Build history of the part. All positions in model axes, mm. A direction names the side the tool comes from. Give positions to 0.01 mm unless a question says otherwise; leave off trailing zeros. Write each loop counter-clockwise with the first axis right and the second up, starting at its lowest first coordinate (ties: lowest second). Pieces come first, ordered by that corner, then holes. Notation, with made-up numbers: (4, -31) -> (42, -31) arc R24 cw to (42, 5) -> close; hole circle Ø6 at (-29, 76.5). An arc over 180 degrees is marked (long way). Put each result on its own line as item: value.
Autodesk Inventor part; units mm, degrees
ref_plane "YZ Plane" through (0, 0, 0) normal (1, 0, 0) x (0, 1, 0)
ref_plane "XZ Plane" through (0, 0, 0) normal (0, 1, 0) x (-1, 0, 0)
ref_plane "XY Plane" through (0, 0, 0) normal (0, 0, 1) x (1, 0, 0)
sketch "Sketch1" plane through (0, 0, 0) normal (0, 0, 1) x (1, 0, 0)
  line L0 (65, -65) -> (-65, -65)
  line L1 (-65, -65) -> (-65, 65)
  line L2 (-65, 65) -> (65, 65)
  line L3 (65, 65) -> (65, -65)
  line L4 (65, -65) -> (-65, 65) construction
  line L5 (-65, -65) -> (65, 65) construction
  circle A0 centre (0, 0) radius 72.5 construction
  circle A1 centre (-51.2652, 51.2652) radius 4.5
  circle A2 centre (51.2652, 51.2652) radius 4.5
  line L6 (-65, 0) -> (65, 0) construction
  circle A3 centre (-51.2652, -51.2652) radius 4.5
  circle A4 centre (51.2652, -51.2652) radius 4.5
  dimension "d0" = 130
  dimension "d1" = 130
  dimension "d2" = 145
  dimension "d3" = 9
  dimension "d4" = 9
extrude "Extrusion1" add sketch "Sketch1" along normal blind 10
fillet "Fillet1" radius 5 4 edges at (-65, -65, 5) (65, -65, 5) (65, 65, 5) (-65, 65, 5)
sketch "Sketch2" plane through (0, 0, 10) normal (0, 0, 1) x (1, 0, 0)
  circle A0 centre (0, 0) radius 55
  circle A1 centre (0, 0) radius 54
  dimension "d8" = 110
extrude "Extrusion2" add sketch "Sketch2" along normal blind 5
sketch "Sketch3" plane through (0, 0, 10) normal (0, 0, 1) x (1, 0, 0)
  circle A0 centre (0, 0) radius 15
  line L0 (0, 0) -> (24.7487, -24.7487) construction
  line L1 (0, 0) -> (35, 0) construction
  line L2 (0, 0) -> (-24.7487, -24.7487) construction
  line L3 (0, 0) -> (35, 0) construction
  line L4 (0, 0) -> (24.7487, 24.7487) construction
  line L5 (0, 0) -> (-24.7487, 24.7487) construction
  line L6 (0.7071, 0.7071) -> (-24.0416, 25.4558) construction
  line L7 (37.8235, -36.4093) -> (25.4457, -24.0315)
  line L8 (36.4093, -37.8235) -> (24.0315, -25.4457)
  line L9 (-36.4093, -37.8235) -> (-24.0315, -25.4457)
  line L10 (-37.8235, -36.4093) -> (-25.4457, -24.0315)
  line L11 (-25.4457, 24.0315) -> (-37.8235, 36.4093)
  line L12 (-24.0315, 25.4457) -> (-36.4093, 37.8235)
  line L13 (-25.4457, 24.0315) -> (-25.4558, 24.0416)
  line L14 (-24.0315, 25.4457) -> (-24.0416, 25.4558)
  line L15 (-25.4457, 24.0315) -> (-25.4558, 24.0416)
  line L16 (36.4093, 37.8235) -> (24.0315, 25.4457)
  line L17 (37.8235, 36.4093) -> (25.4457, 24.0315)
  arc A1 (-24.0315, -25.4457) -> (24.0315, -25.4457) centre (0, 0) ccw
  arc A2 (-25.4457, 24.0315) -> (-25.4457, -24.0315) centre (0, 0) ccw
  arc A3 (25.4457, -24.0315) -> (25.4457, 24.0315) centre (0, 0) ccw
  arc A4 (24.0315, 25.4457) -> (-24.0315, 25.4457) centre (0, 0) ccw
  arc A5 (-36.4093, -37.8235) -> (36.4093, -37.8235) centre (0, 0) ccw
  arc A6 (-37.8235, 36.4093) -> (-37.8235, -36.4093) centre (0, 0) ccw
  arc A7 (37.8235, -36.4093) -> (37.8235, 36.4093) centre (0, 0) ccw
  arc A8 (36.4093, 37.8235) -> (-36.4093, 37.8235) centre (0, 0) ccw
  circle A9 centre (0, 0) radius 54
  dimension "d12" = 30
  dimension "d14" = 45
  dimension "d15" = 135
extrude "Extrusion3" add sketch "Sketch3" along normal blind 5
sketch "Sketch4" plane through (0, 0, 0) normal (0, 1, 0) x (-1, 0, 0)
  line L0 (15, 15) -> (15, 10)
  line L1 (15, 10) -> (15, 15)
  line L2 (0, 15) -> (11, 15) construction
  line L3 (15, 15) -> (13, 15)
  line L4 (13, 15) -> (13, 20)
  line L5 (11, 16) -> (11, 67) construction
  line L6 (60, 10) -> (65, 10) construction
  line L7 (13, 20) -> (11, 20)
  line L8 (11, 67) -> (11, 20)
  line L9 (11, 67) -> (0, 67)
  line L10 (0, 67) -> (0, 10)
  line L11 (15, 10) -> (0, 10)
  line L12 (0, -13.4) -> (0, 80.4)
  point P0 (0, 0)
  dimension "d18" = 11
  dimension "d19" = 2
  dimension "d20" = 5
  dimension "d21" = 57
revolve "Revolution1" add sketch "Sketch4" angle 360 about axis through (0, 0, -10) along (0, 0, 1)
sketch "Sketch5" plane through (0, 0, 0) normal (0, 0, -1) x (-1, 0, 0)
  line L0 (-45.7652, 55.7652) -> (45.7652, 55.7652)
  line L1 (55.7652, 45.7652) -> (55.7652, -45.7652)
  line L2 (45.7652, -55.7652) -> (-45.7652, -55.7652)
  line L3 (-55.7652, -45.7652) -> (-55.7652, 45.7652)
  line L4 (-55.7652, 55.7652) -> (55.7652, -55.7652) construction
  line L5 (55.7652, 55.7652) -> (-55.7652, -55.7652) construction
  line L6 (55.7652, -55.7652) -> (55.7652, -45.7652) construction
  line L7 (55.7652, -45.7652) -> (50.7652, -45.7652)
  line L8 (45.7652, -55.7652) -> (45.7652, -50.7652)
  arc A0 (50.7652, -45.7652) -> (45.7652, -50.7652) centre (50.7652, -50.7652) ccw
  line L9 (0, 0) -> (0, -55.7652) construction
  line L10 (0, 0) -> (-55.7652, 0) construction
  line L11 (-55.7652, -45.7652) -> (-50.7652, -45.7652)
  line L12 (-45.7652, -55.7652) -> (-45.7652, -50.7652)
  arc A1 (-45.7652, -50.7652) -> (-50.7652, -45.7652) centre (-50.7652, -50.7652) ccw
  line L13 (55.7652, 45.7652) -> (50.7652, 45.7652)
  line L14 (45.7652, 55.7652) -> (45.7652, 50.7652)
  arc A2 (45.7652, 50.7652) -> (50.7652, 45.7652) centre (50.7652, 50.7652) ccw
  line L15 (-45.7652, 55.7652) -> (-45.7652, 50.7652)
  arc A3 (-50.7652, 45.7652) -> (-45.7652, 50.7652) centre (-50.7652, 50.7652) ccw
  line L16 (-55.7652, 45.7652) -> (-50.7652, 45.7652)
  point P0 (45.7652, -45.7652)
  dimension "d23" = 10
  dimension "d24" = 5
extrude "Extrusion4" add sketch "Sketch5" along normal blind 201
sketch "Sketch6" plane through (0, 0, -201) normal (0, 0, -1) x (-1, 0, 0)
  circle A0 centre (0, 0) radius 30
  dimension "d27" = 60
extrude "Extrusion5" add sketch "Sketch6" along normal blind 30
properties part number "SERVOMOTOR-2.3KWv1" material "Iron, Cast"
1) Pin check, flat tips, straight feed: pin 1 (6 mm diameter, centred on x = -46, y = 37, fed in from +Z); pin 2 (3 mm diameter, centred on x = 45, y = 21, fed in from -Z); pin 3 (1 mm diameter, centred on x = 42.5, z = -124.5, fed in from -Y). Stop position of each tip, or through.
Filled sheet:
pin 1: z = 10
pin 2: z = -201
pin 3: y = -55.77
2) Slice it at D-D (y = 18). Write the cut outline in (x, z), plus the area to 3 significant figures.
Filled sheet:
outline: (-65, 0) -> (-55.77, 0) -> (-55.77, -201) -> (-24, -201) -> (-24, -231) -> (24, -231) -> (24, -201) -> (55.77, -201) -> (55.77, 0) -> (65, 0) -> (65, 10) -> (51.97, 10) -> (51.97, 15) -> (49.32, 15) -> (49.32, 10) -> (30.02, 10) -> (30.02, 15) -> (-30.02, 15) -> (-30.02, 10) -> (-49.32, 10) -> (-49.32, 15) -> (-51.97, 15) -> (-51.97, 10) -> (-65, 10) -> close
area: 25,500 mm2
3) Wall check: L1, parallel to Y at x = 49, z = 5; L2, parallel to Y at x = -55, z = -124; L3, parallel to X at y = 7, z = -145. Give the ranges that are in metal, low to high.
Filled sheet:
L1: -65 to -55.15, -47.38 to 47.38, 55.15 to 65
L2: -45.77 to 45.77
L3: -55.77 to 55.77
4) Tool access for faces 1 (the flat face through (-65, -1, 5)), 2 (the flat face through (1, -65, 5)), 3 (the flat face through (31.721, -30.307, 12.465)), 4 (the flat face through (55.765, -1, -99)), 5 (the cylindrical face through (29.97, -1.32, -215.79)): list every direction of +Z, -Z, +X, -X, +Y, -Y with a clear straight run to the whole face (end or side of a thin tool).
Filled sheet:
face 1: +Z, -Z, -X, +Y, -Y
face 2: +Z, -Z, +X, -X, -Y
face 3: +Z
face 4: -Z, +X, +Y, -Y
face 5: -Z
5) Slice it at B-B (z = -142.5). Write the cut outline in (x, y).
Filled sheet:
outline: (-55.77, -45.77) -> (-50.77, -45.77) arc R5 cw to (-45.77, -50.77) -> (-45.77, -55.77) -> (45.77, -55.77) -> (45.77, -50.77) arc R5 cw to (50.77, -45.77) -> (55.77, -45.77) -> (55.77, 45.77) -> (50.77, 45.77) arc R5 cw to (45.77, 50.77) -> (45.77, 55.77) -> (-45.77, 55.77) -> (-45.77, 50.77) arc R5 cw to (-50.77, 45.77) -> (-55.77, 45.77) -> close
